```python
from build123d import *

# Parameters (mm, degrees)
EXTRUDE_1_DEPTH = 104
SKETCH_1_23_R   = 1.5
EXTRUDE_2_DEPTH = 4
EXTRUDE_START   = 100
SKETCH_1_24_R   = 1.5
EXTRUDE_3_DEPTH = 4
FILLET_1_R      = 1


with BuildPart() as part:
    # 草图1 → 凸台-拉伸1 (new body)
    with BuildSketch(Plane.XY):
        with BuildLine():
            Line((17.75, -10.5), (17.75, -0.328219619))
            ThreePointArc((17.75, -0.328219619), (11.588859881, -6.801694776), (2.75, -8.120817283))
            Line((2.75, -8.120817283), (2.75, -19))
            Line((2.75, -19), (9.25, -19))
            Line((9.25, -19), (9.25, -14))
            ThreePointArc((9.25, -14), (10.275126266, -11.525126266), (12.75, -10.5))
            Line((12.75, -10.5), (17.75, -10.5))
        make_face()
    extrude(amount=EXTRUDE_1_DEPTH)

    # 草图1<23> → 凸台-拉伸2 (add)
    with BuildSketch(Plane.XY):
        with BuildLine():
            Line((17.75, -14), (17.75, -10.5))
            Line((17.75, -10.5), (12.75, -10.5))
            ThreePointArc((12.75, -10.5), (10.275126266, -11.525126266), (9.25, -14))
            Line((9.25, -14), (9.25, -19))
            Line((9.25, -19), (12.75, -19))
            ThreePointArc((12.75, -19), (16.285533906, -17.535533906), (17.75, -14))
        make_face()
        with Locations((12.75, -14)):
            Circle(SKETCH_1_23_R, mode=Mode.SUBTRACT)
    extrude(amount=EXTRUDE_2_DEPTH)

    # 草图1<24> → 凸台-拉伸3 (add)
    with BuildSketch(Plane.XY.offset(EXTRUDE_START)):
        with BuildLine():
            Line((17.75, -14), (17.75, -10.5))
            Line((17.75, -10.5), (12.75, -10.5))
            ThreePointArc((12.75, -10.5), (10.275126266, -11.525126266), (9.25, -14))
            Line((9.25, -14), (9.25, -19))
            Line((9.25, -19), (12.75, -19))
            ThreePointArc((12.75, -19), (16.285533906, -17.535533906), (17.75, -14))
        make_face()
        with Locations((12.75, -14)):
            Circle(SKETCH_1_24_R, mode=Mode.SUBTRACT)
    extrude(amount=EXTRUDE_3_DEPTH)

    # 圆角1
    fillet_1_edges = [part.edges().sort_by_distance(p)[0] for p in [
        (2.75, -19, 52),
        (2.75, -8.120817283, 52),
        (17.75, -0.328219619, 52),
    ]]
    fillet(fillet_1_edges, radius=FILLET_1_R)


solid = part.part
```
Design review of the part built by this model. Coordinates are the model's own, in mm. A direction names the side the tool comes from. Round coordinates to 2 decimals unless told otherwise and drop trailing zeros. Write each loop counter-clockwise with the first axis right and the second up, starting at its lowest first coordinate (ties: lowest second). Pieces come first, ordered by that corner, then holes.
Item 1: We need section C-C on x = 7.5. Write out the cut boundary in (y, z).
Item 2: The part is to be moulded in two halves that separate along X. For faces 1 (the cylindrical face through (16.25, -17.57, 101.97)), 2 (the cylindrical face through (10.64, -7.25, 51.27)), 3 (the cylindrical face through (17.1, -2.9, 52.7)), say which applies: +X half, -X half, draft (parallel to the pull), parting line (faces both ways), or undercut.
Item 3: For probe 1 along Z at (x, y) = (11.75, -17); probe 2 along Y at (x, z) = (6, 94.5); probe 3 along X at (y, z) = (-16.5, 28), list the stretches that pass through material, from the lowest coordinate up.
Item 4: We need section D-D on y = -7. Write out the cut boundary in (x, z), and give its area (3 significant figures).
Item 5: Clearance check with flat-ended pins moving along their axes: pin 1 Ø4 at (x, z) = (15, 56.5) entering from -Y; pin 2 Ø2 at (x, z) = (12, 23.5) entering from +Y; pin 3 Ø8 at (x, z) = (10, 88.5) entering from +Y. State where each tip first meets the part, or that it passes through.
Item 6: For faces 4 (the flat face through (13, -16, 4)), 5 (the flat face through (2.75, -14, 51)), list the 3-axis set-ups (+Z, -Z, +X, -X, +Y, -Y) from which the entire face can be reached by the end or side of a thin tool; tool diameter is ignored.
Item 7: We need section A-A on z = 16. Write out the cut boundary in (x, y).
Item 8: We need section B-B on y = -16.75. Write out the cut boundary in (x, z).
Returned:
1. outline: (-19, 0) - (-8.16, 0) - (-8.16, 104) - (-19, 104) - close
2. face 1: +X half
2. face 2: undercut
2. face 3: parting line
3. probe 1: z = 0 to 4, 100 to 104
3. probe 2: y = -19 to -8.33
3. probe 3: x = 2.75 to 9.25
4. outline: (11.19, 0) - (17.75, 0) - (17.75, 104) - (11.19, 104) - close
4. area: 682 mm2
5. pin 1: stops at y = -10.5
5. pin 2: stops at y = -5.96
5. pin 3: stops at y = -5.21
6. face 4: +X, -Y
6. face 5: +Z, -Z, -X, +Y, -Y
7. outline: (2.75, -18) arc R1 ccw to (3.75, -19) - (9.25, -19) - (9.25, -14) arc R3.5 cw to (12.75, -10.5) - (17.75, -10.5) - (17.75, -3.84) arc R1 ccw to (15.97, -3.21) arc R13.75 cw to (3.85, -8.28) arc R1 ccw to (2.75, -9.27) - close
8. outline: (2.75, 0) - (16.93, 0) - (16.93, 4) - (9.25, 4) - (9.25, 100) - (16.93, 100) - (16.93, 104) - (2.75, 104) - close
